```python
from build123d import *

# Parameters (mm, degrees)
SKETCH3_W = 7.62
SKETCH3_H = 1.5875
FILLET1_R = 0.508


with BuildPart() as part:
    # Sweep1: sweep along a path in Sketch2
    with BuildLine(Plane(origin=(12.652967073, 0, 0), x_dir=(0, 0, -1), z_dir=(1, 0, 0))) as sweep1_path:
        Line((0.8255, -25.883657999), (0.8255, 29.996342001))
        ThreePointArc((0.8255, 29.996342001), (0.081551224, 31.792393225), (-1.7145, 32.536342001))
        Line((-1.7145, 32.536342001), (-9.525, 32.536342001))
        ThreePointArc((-9.525, 32.536342001), (-9.930637017, 32.510323362), (-10.329625768, 32.432693881))
        Line((-10.329625768, 32.432693881), (-34.489200615, 26.103423505))
        ThreePointArc((-34.489200615, 26.103423505), (-35.683232492, 25.399721391), (-36.330095218, 24.173965541))
        Line((-36.330095218, 24.173965541), (-37.665372012, 17.886106714))
        ThreePointArc((-37.665372012, 17.886106714), (-37.691319269, 17.72213092), (-37.7, 17.556342001))
        Line((-37.7, 17.556342001), (-37.7, -13.443657999))
        ThreePointArc((-37.7, -13.443657999), (-37.691319269, -13.609446919), (-37.665372012, -13.773422712))
        Line((-37.665372012, -13.773422712), (-36.330095218, -20.061281539))
        ThreePointArc((-36.330095218, -20.061281539), (-35.683232492, -21.287037389), (-34.489200615, -21.990739503))
        Line((-34.489200615, -21.990739503), (-10.329625768, -28.320009879))
        ThreePointArc((-10.329625768, -28.320009879), (-9.930637017, -28.39763936), (-9.525, -28.423657999))
        Line((-9.525, -28.423657999), (-1.7145, -28.423657999))
        ThreePointArc((-1.7145, -28.423657999), (0.081551224, -27.679709223), (0.8255, -25.883657999))
    # Sketch3 → Sweep1 (sweep)
    with BuildSketch(Plane(origin=(0, 0, 0), x_dir=(1, 0, 0), z_dir=(0, 1, 0))):
        with Locations((12.652967073, 1.61925)):
            Rectangle(SKETCH3_W, SKETCH3_H)
    sweep(path=sweep1_path.line)

    # Fillet1
    fillet1_edges = [part.edges().sort_by_distance(p)[0] for p in [
        (16.462967073, -26.691050632, 22.811726076),
        (8.842967073, -26.691050632, 22.811726076),
        (8.842967073, -25.155374691, 22.409413191),
        (16.462967073, -21.287037389, 35.683232492),
        (16.462967073, -22.382899508, 36.8318153),
        (8.842967073, -22.382899508, 36.8318153),
        (8.842967073, -21.287037389, 35.683232492),
        (16.462967073, -16.917352126, 36.997733615),
        (16.462967073, -17.247116838, 38.550605627),
        (8.842967073, -17.247116838, 38.550605627),
        (8.842967073, -16.917352126, 36.997733615),
        (16.462967073, -13.609446919, 37.691319269),
        (16.462967073, -13.775235838, 39.270138538),
        (8.842967073, -13.775235838, 39.270138538),
        (16.462967073, 2.056342001, -0.8255),
        (8.842967073, -13.609446919, 37.691319269),
        (16.462967073, 2.056342001, 37.7),
        (16.462967073, 2.056342001, 39.2875),
        (8.842967073, 2.056342001, 39.2875),
        (8.842967073, 2.056342001, 37.7),
        (16.462967073, 2.056342001, -2.413),
        (16.462967073, 17.72213092, 37.691319269),
        (16.462967073, 17.88791984, 39.270138538),
        (8.842967073, 17.88791984, 39.270138538),
        (8.842967073, 17.72213092, 37.691319269),
        (16.462967073, 21.030036127, 36.997733615),
        (16.462967073, 21.35980084, 38.550605627),
        (8.842967073, 21.35980084, 38.550605627),
        (8.842967073, 2.056342001, -2.413),
        (8.842967073, 21.030036127, 36.997733615),
        (16.462967073, 25.399721391, 35.683232492),
        (16.462967073, 26.49558351, 36.8318153),
        (8.842967073, 26.49558351, 36.8318153),
        (8.842967073, 25.399721391, 35.683232492),
        (16.462967073, 29.268058693, 22.409413191),
        (16.462967073, 30.803734633, 22.811726076),
        (8.842967073, 30.803734633, 22.811726076),
        (8.842967073, 29.268058693, 22.409413191),
        (16.462967073, 32.510323362, 9.930637017),
        (8.842967073, 2.056342001, -0.8255),
        (16.462967073, 34.084814042, 10.133455526),
        (8.842967073, 34.084814042, 10.133455526),
        (8.842967073, 32.510323362, 9.930637017),
        (16.462967073, 32.536342001, 5.61975),
        (16.462967073, 34.123842001, 5.61975),
        (8.842967073, 34.123842001, 5.61975),
        (8.842967073, 32.536342001, 5.61975),
        (16.462967073, 31.792393225, -0.081551224),
        (16.462967073, 32.91492524, -1.204083239),
        (8.842967073, 32.91492524, -1.204083239),
        (8.842967073, 31.792393225, -0.081551224),
        (16.462967073, 2.056342001, -0.8255),
        (16.462967073, 2.056342001, -2.413),
        (8.842967073, 2.056342001, -2.413),
        (8.842967073, 2.056342001, -0.8255),
        (16.462967073, -27.679709223, -0.081551224),
        (16.462967073, -28.802241238, -1.204083239),
        (8.842967073, -28.802241238, -1.204083239),
        (8.842967073, -27.679709223, -0.081551224),
        (16.462967073, -28.423657999, 5.61975),
        (16.462967073, -30.011157999, 5.61975),
        (8.842967073, -30.011157999, 5.61975),
        (8.842967073, -28.423657999, 5.61975),
        (16.462967073, -28.39763936, 9.930637017),
        (16.462967073, -29.97213004, 10.133455526),
        (8.842967073, -29.97213004, 10.133455526),
        (8.842967073, -28.39763936, 9.930637017),
        (16.462967073, -25.155374691, 22.409413191),
    ]]
    fillet(fillet1_edges, radius=FILLET1_R)


solid = part.part
```
Verification items for the finished model (mm, model axes). A direction names the side the tool comes from. Give positions to 0.01 mm unless a question says otherwise; leave off trailing zeros. Order: outer loops, then holes, each group sorted by start corner. A loop starts at its lowest first (then second) coordinate and runs counter-clockwise, first axis right, second up. Notation, with made-up numbers: (88.5, -25.75) -> (146.5, -25.75) arc R17 ccw to (146.5, -4.75) -> close; hole circle Ø5 at (72, 54.25). An arc over 180 degrees is marked (long way). One line per item, written item: value.
(1) Gauge pin test, flat ends, axial feed: pin 1 (2 mm diameter, centred on x = 13.5, z = 16.5, fed in from -Y); pin 2 (3 mm diameter, centred on x = 15, z = 32.5, fed in from -Y). Record the tip position at first contact, or that the pin passes through.
Final values:
pin 1: y = -28.61
pin 2: y = -24.55
(2) Draft check along Z on faces 1 (the face through (8.843, 20.9, 37.9)), 2 (the face through (16.32, 21.02, 37.16)), 3 (the face through (12.607, 34.086, 10.125)), 4 (the face through (12.607, 29.224, 22.579)). Enter one of: pulls with the +Z half, pulls with the -Z half, needs draft (parallel to the pull), parting line crosses it, or undercut.
Final values:
face 1: needs draft
face 2: undercut
face 3: pulls with the +Z half
face 4: undercut
(3) Tool access check on faces 5 (the face through (8.99, 29.37, 22.62)), 6 (the face through (13, 34.124, 6)), 7 (the face through (13, 2, -0.826)). Record the directions out of +Z, -Z, +X, -X, +Y, -Y that give a thin tool (end or side, any length) a straight path to the whole face; none if there is none.
Final values:
face 5: -X
face 6: +Z, -Z, +X, -X, +Y
face 7: +X, -X
(4) Sectioned sample at A-A on z = 7.5. Record the cut outline in (x, y), then the cut area to 3 significant figures.
Final values:
outline: (8.84, -29.5) arc R0.51 ccw to (9.35, -30.01) -> (15.95, -30.01) arc R0.51 ccw to (16.46, -29.5) -> (16.46, -28.93) arc R0.51 ccw to (15.95, -28.42) -> (9.35, -28.42) arc R0.51 ccw to (8.84, -28.93) -> close; (8.84, 33.04) arc R0.51 ccw to (9.35, 32.54) -> (15.95, 32.54) arc R0.51 ccw to (16.46, 33.04) -> (16.46, 33.62) arc R0.51 ccw to (15.95, 34.12) -> (9.35, 34.12) arc R0.51 ccw to (8.84, 33.62) -> close
area: 23.8 mm^2
(5) Scan lines: line 1 along Z through (x, y) = (12, 16.5); line 2 along Y through (x, z) = (13.5, 5); line 3 along Y through (x, z) = (9.5, 22). Record each from-to range of solid material in increasing order. Write a range as [from, to].
Final values:
line 1: [-2.41, -0.83], [37.7, 39.29]
line 2: [-30.01, -28.42], [32.54, 34.12]
line 3: [-26.9, -25.26], [29.38, 31.02]
